Design review of the part built by this model. Coordinates are the model's own, in mm. Round coordinates to 2 decimals unless told otherwise and drop trailing zeros. Order: outer loops, then holes, each group sorted by start corner. A loop starts at its lowest first (then second) coordinate and runs counter-clockwise, first axis right, second up. Notation, with made-up numbers: (-39.5, -26.75) - (11.5, -26.75) arc R28 ccw to (11.5, -4.75) - close; hole circle Ø4 at (-10, -1). An arc over 180 degrees is marked (long way). Use CSV: the item, a comma, the result in double quotes.
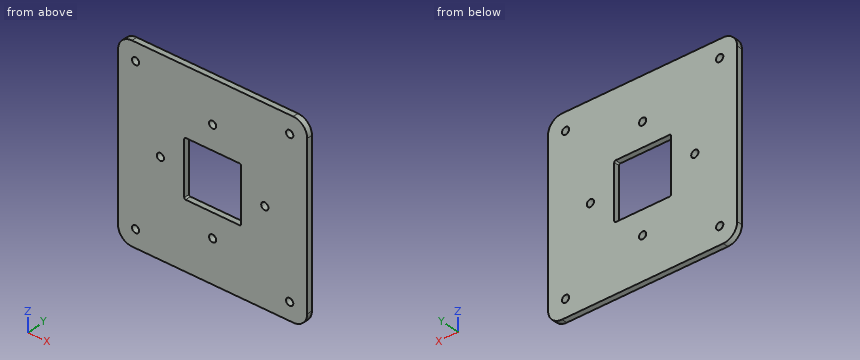
from build123d import *

# Parameters (mm, degrees)
SKETCH1_W           = 135
SKETCH1_H           = 135
BOSS_EXTRUDE1_DEPTH = 4
CUT_EXTRUDE1_DEPTH  = 96.543183954
SKETCH5_R           = 2.58
CUT_EXTRUDE2_DEPTH  = 96.543183954
SKETCH6_R           = 2.58
CUT_EXTRUDE3_DEPTH  = 96.543183954
FILLET1_R           = 10


with BuildPart() as part:
    # Sketch1 → Boss-Extrude1 (new body)
    with BuildSketch(Plane(origin=(0, 0, 0), x_dir=(1, 0, 0), z_dir=(0, 1, 0))):
        Rectangle(SKETCH1_W, SKETCH1_H)
    extrude(amount=BOSS_EXTRUDE1_DEPTH)

    # Sketch4 → Cut-Extrude1 (cut, through all)
    with BuildSketch(Plane(origin=(0, 4, 0), x_dir=(1, 0, 0), z_dir=(0, 1, 0))):
        with BuildLine():
            Line((-19.25, 20.25), (19.25, 20.25))
            ThreePointArc((19.25, 20.25), (19.957106781, 19.957106781), (20.25, 19.25))
            Line((20.25, 19.25), (20.25, -19.25))
            ThreePointArc((20.25, -19.25), (19.957106781, -19.957106781), (19.25, -20.25))
            Line((19.25, -20.25), (-19.25, -20.25))
            ThreePointArc((-19.25, -20.25), (-19.957106781, -19.957106781), (-20.25, -19.25))
            Line((-20.25, -19.25), (-20.25, 19.25))
            ThreePointArc((-20.25, 19.25), (-19.957106781, 19.957106781), (-19.25, 20.25))
        make_face()
    extrude(amount=-CUT_EXTRUDE1_DEPTH, mode=Mode.SUBTRACT)

    # Sketch5 → Cut-Extrude2 (cut, through all)
    with BuildSketch(Plane(origin=(0, 4, 0), x_dir=(1, 0, 0), z_dir=(0, 1, 0))):
        with Locations(Location((-37.25, 0, 0), (0, 0, 270))):
            Circle(SKETCH5_R)
        with Locations(Location((0, 37.25, 0), (0, 0, 270))):
            Circle(SKETCH5_R)
        with Locations(Location((37.25, 0, 0), (0, 0, 270))):
            Circle(SKETCH5_R)
        with Locations(Location((0, -37.25, 0), (0, 0, 270))):
            Circle(SKETCH5_R)
    extrude(amount=-CUT_EXTRUDE2_DEPTH, mode=Mode.SUBTRACT)

    # Sketch6 → Cut-Extrude3 (cut, through all)
    with BuildSketch(Plane(origin=(0, 4, 0), x_dir=(1, 0, 0), z_dir=(0, 1, 0))):
        with Locations(Location((-55, 55, 0), (0, 0, 270))):
            Circle(SKETCH6_R)
        with Locations(Location((55, 55, 0), (0, 0, 270))):
            Circle(SKETCH6_R)
        with Locations(Location((55, -55, 0), (0, 0, 270))):
            Circle(SKETCH6_R)
        with Locations(Location((-55, -55, 0), (0, 0, 270))):
            Circle(SKETCH6_R)
    extrude(amount=-CUT_EXTRUDE3_DEPTH, mode=Mode.SUBTRACT)

    # Fillet1
    fillet1_edges = [part.edges().sort_by_distance(p)[0] for p in [
        (67.5, 2, 67.5),
        (-67.5, 2, 67.5),
        (-67.5, 2, -67.5),
        (67.5, 2, -67.5),
    ]]
    fillet(fillet1_edges, radius=FILLET1_R)


solid = part.part
1) We need section B-B (y = 2.25). Give the number of separate pieces and of enclosed holes in the cut face, then the cut area to 3 significant figures.
Data:
separate pieces,"1"
enclosed holes,"9"
area,"16,300 mm2"
2) We need section A-A (x = 37.25). Give the boundary of the cut face in (y, z), then the cut area to 3 significant figures.
Data:
outline,"(0, -67.5) - (4, -67.5) - (4, -2.58) - (0, -2.58) - close; (0, 2.58) - (4, 2.58) - (4, 67.5) - (0, 67.5) - close"
area,"519 mm2"
3) We need section D-D (x = -55). Give the boundary of the cut face in (y, z).
Data:
outline,"(0, -67.5) - (4, -67.5) - (4, -57.58) - (0, -57.58) - close; (0, -52.42) - (4, -52.42) - (4, 52.42) - (0, 52.42) - close; (0, 57.58) - (4, 57.58) - (4, 67.5) - (0, 67.5) - close"
4) To check wall thickness, follow L1, parallel to X at y = 0.8, z = -15; L2, parallel to X at y = 2.4, z = 0; L3, parallel to X at y = 3.1, z = -55. State the ranges of each line that lie inside material, in increasing order. Write a range as from..to.
Data:
L1,"x = -67.5..-20.25, 20.25..67.5"
L2,"x = -67.5..-39.83, -34.67..-20.25, 20.25..34.67, 39.83..67.5"
L3,"x = -67.5..-57.58, -52.42..52.42, 57.58..67.5"
5) We need section C-C (z = -37.25). Give the boundary of the cut face in (x, y).
Data:
outline,"(-67.5, 0) - (-2.58, 0) - (-2.58, 4) - (-67.5, 4) - close; (2.58, 0) - (67.5, 0) - (67.5, 4) - (2.58, 4) - close"
